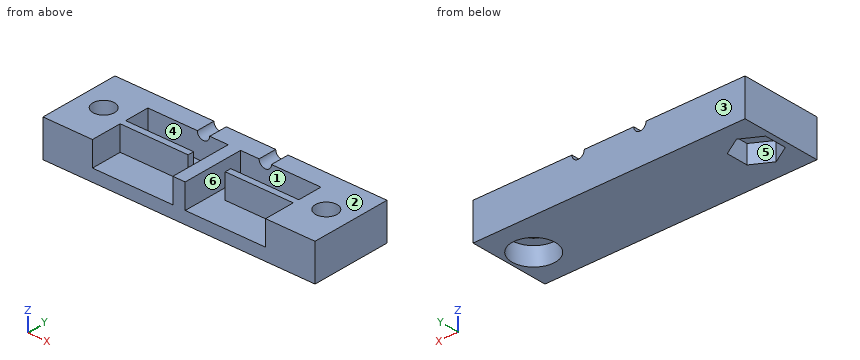
from build123d import *

# Parameters (mm, degrees)
PAD_DEPTH       = 4
SKETCH001_R     = 1
POCKET_DEPTH    = 5
SKETCH002_W     = 44
SKETCH002_H     = 13
PAD001_DEPTH    = 2
SKETCH004_R     = 3.5
POCKET001_DEPTH = 3
SKETCH005_R     = 1.75
POCKET002_DEPTH = 5


with BuildPart() as part:
    # Sketch → Pad (new body)
    with BuildSketch(Plane.XY):
        Polygon((8, 10), (8, 6), (19, 6), (19, 5), (8, 5), (8, 0), (0, 0), (0, 13), (44, 13), (44, 0), (36, 0), (36, 5), (25, 5), (25, 6), (36, 6), (36, 10), (23, 10), (23, 0), (21, 0), (21, 10), align=None)
    extrude(amount=PAD_DEPTH)

    # Sketch001 → Pocket (cut)
    with BuildSketch(Plane(origin=(0, 13, 0), x_dir=(-1, 0, 0), z_dir=(0, 1, 0))):
        with Locations((-27, 4)):
            Circle(SKETCH001_R)
        with Locations((-17, 4)):
            Circle(SKETCH001_R)
    extrude(amount=-POCKET_DEPTH, mode=Mode.SUBTRACT)

    # Sketch002 → Pad001 (new body)
    with BuildSketch(Plane(origin=(0, 0, 0), x_dir=(1, 0, 0), z_dir=(0, 0, -1))):
        with Locations((22, -6.5)):
            Rectangle(SKETCH002_W, SKETCH002_H)
    extrude(amount=PAD001_DEPTH)

    # Sketch004 → Pocket001 (cut)
    with BuildSketch(Plane(origin=(0, 0, -2), x_dir=(1, 0, 0), z_dir=(0, 0, -1))):
        with Locations((40, -6.5)):
            Circle(SKETCH004_R)
        Polygon((0.9, -8.289786), (0.9, -4.710214), (4, -2.920428), (7.1, -4.710214), (7.1, -8.289786), (4, -10.079572), align=None)
    extrude(amount=-POCKET001_DEPTH, mode=Mode.SUBTRACT)

    # Sketch005 → Pocket002 (cut)
    with BuildSketch(Plane.XY.offset(4)):
        with Locations((4, 6.5)):
            Circle(SKETCH005_R)
        with Locations((40, 6.5)):
            Circle(SKETCH005_R)
    extrude(amount=-POCKET002_DEPTH, mode=Mode.SUBTRACT)


solid = part.part
Source: CAD feature listing. Evaluate the final solid. Frame: model axes, mm. Face numbers are marked on the shaded views. A direction names the side the tool comes from. Round coordinates to 2 decimals unless told otherwise and drop trailing zeros. Write each loop counter-clockwise with the first axis right and the second up, starting at its lowest first coordinate (ties: lowest second). Pieces come first, ordered by that corner, then holes. Notation, with made-up numbers: M 62,43 L 82,43 A19 ccw 82,63 Z; hole C -17,31 d2. An arc over 180 degrees is marked long. One line per item, written item: value. Start each with the question number.
Item 1: Pin query (flat end, axial travel): pin 1 (3 mm diameter, centred on x = 26.5, z = 2.5, fed in from -Y). Return the tip coordinate at first contact, or that it passes through.
Item 2: Section query D-D (z = 3.6). State how many separate pieces and enclosed holes the cut face has, plus the area to 3 significant figures.
Item 3: Section query B-B (x = 40). Return the cut outline in (y, z), plus the area to 3 significant figures.
Item 4: Section query C-C (y = 6.5). Return the cut outline in (x, z), plus the area to 3 significant figures.
Item 5: Set-up query: the marked faces 4, 5 and 6. Return all of +Z, -Z, +X, -X, +Y, -Y with unobstructed straight access to the full face (end or side cutting, diameter ignored); none if empty.
Item 6: Section query A-A (z = -0.5). Return the cut outline in (x, y), plus the area to 3 significant figures.
Item 7: Ray query, L1, parallel to X at y = 6.5, z = -1.4; L2, parallel to X at y = 3, z = 1.7; L3, parallel to Y at x = 40, z = -1.2. Return the intervals inside material, ascending. Write a range as from..to.
Item 8: Mould query, pull axis Y, two halves, no side actions, for the marked faces 1, 2 and 3. Classes: pulls with the +Y half, pulls with the -Y half, needs draft (parallel to the pull), parting line crosses it, or undercut.
Result set:
1. pin 1: stops at y = 5
2. separate pieces: 3
2. enclosed holes: 2
2. area: 304 mm²
3. outline: M 0,-2 L 3,-2 L 3,1 L 4.75,1 L 4.75,4 L 0,4 Z; M 8.25,1 L 10,1 L 10,-2 L 13,-2 L 13,4 L 8.25,4 Z
3. area: 46.5 mm²
4. outline: M 0,-2 L 0.9,-2 L 0.9,1 L 2.25,1 L 2.25,4 L 0,4 Z; M 5.75,1 L 7.1,1 L 7.1,-2 L 36.5,-2 L 36.5,1 L 38.25,1 L 38.25,4 L 36,4 L 36,0 L 23,0 L 23,4 L 21,4 L 21,0 L 8,0 L 8,4 L 5.75,4 Z; M 41.75,1 L 43.5,1 L 43.5,-2 L 44,-2 L 44,4 L 41.75,4 Z
4. area: 99.4 mm²
5. face 4: +Z
5. face 5: -Z
5. face 6: +Z, -Y
6. outline: M 0,0 L 44,0 L 44,13 L 0,13 Z; hole M 0.9,4.71 L 4,2.92 L 7.1,4.71 L 7.1,8.29 L 4,10.08 L 0.9,8.29 Z; hole C 40,6.5 d7
6. area: 500 mm²
7. L1: x = 0..0.9, 7.1..36.5, 43.5..44
7. L2: x = 0..8, 21..23, 36..44
7. L3: y = 0..3, 10..13
8. face 1: undercut
8. face 2: needs draft
8. face 3: pulls with the +Y half
